Could you check a few things on this drawing? It's one solid part, dimensions in mm from its lowest x, y, z. Give positions to 0.01 mm unless a question says otherwise; leave off trailing zeros. Order: outer loops, then holes, each group sorted by start corner. A loop starts at its lowest first (then second) coordinate and runs counter-clockwise, first axis right, second up. Notation, with made-up numbers: M 85,18 L 103,18 A33 cw 103,56 Z; hole C 48,49.25 d7. An arc over 180 degrees is marked long. Use one line per item in the form item = value.
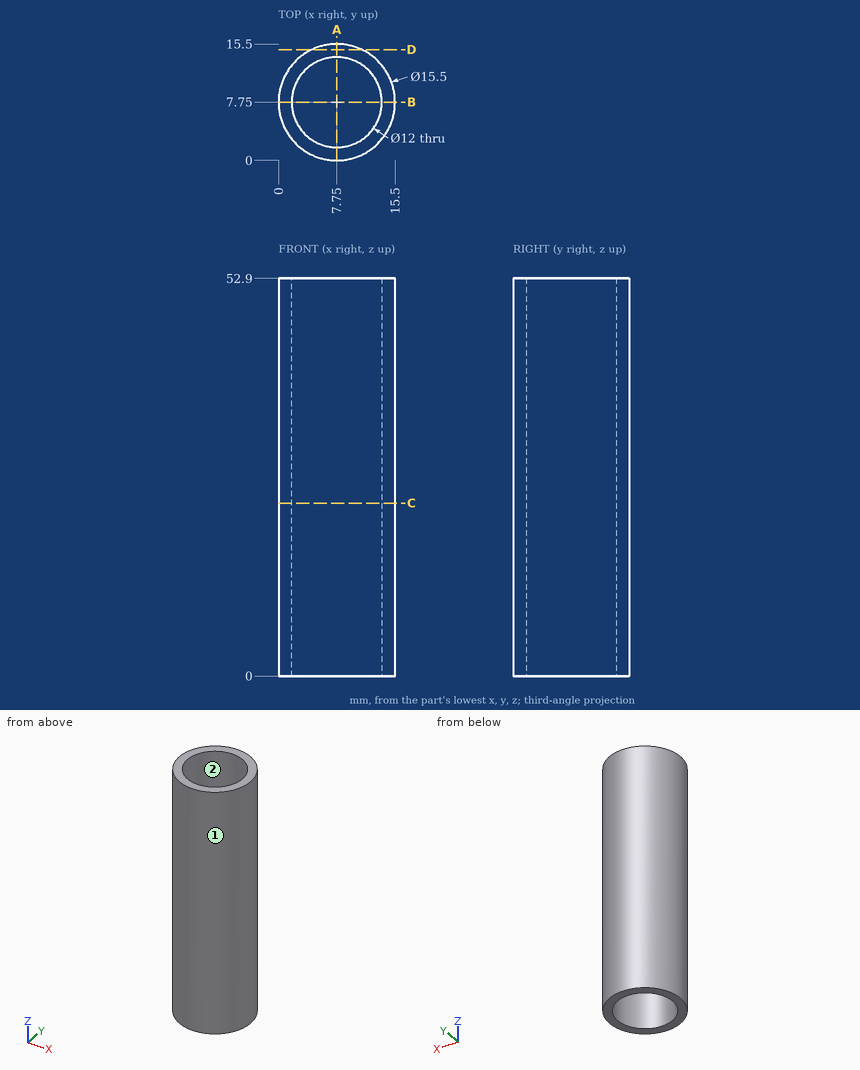
Q1. I want a section at C-C on z = 23. Write out the boundary of the cut face in (x, y).
Found:
outline = C 7.75,7.75 d15.5; hole C 7.75,7.75 d12
Q2. I want a section at D-D on y = 14.75. Write out the boundary of the cut face in (x, z), then the cut area to 3 significant figures.
Found:
outline = M 4.42,0 L 11.08,0 L 11.08,52.9 L 4.42,52.9 Z
area = 352 mm²
Q3. I need wall thicknesses on L1, parallel to Y at x = 7.75, z = 37; L2, parallel to X at y = 5, z = 26. Which ranges of each line are inside material? Lowest first, please.
Found:
L1 = 0 to 1.75, 13.75 to 15.5
L2 = 0.5 to 2.42, 13.08 to 15
Q4. Thinking about a two-plate mould opening in X: for the marked faces 1 and 2, which applies, +X half, -X half, draft (parallel to the pull), parting line (faces both ways), or undercut?
Found:
face_1 = parting line
face_2 = undercut
Q5. I'm going to push flat-ended pins straight in: pin 1 Ø1 at (y, z) = (5, 36) entering from -X; pin 2 Ø1 at (x, z) = (6, 26.5) entering from -Y; pin 3 Ø5 at (y, z) = (2.5, 13.5) entering from -X. Where does each tip first touch, or does it pass through?
Found:
pin_1 = 0.33
pin_2 = 0.1
pin_3 = 0.5
Q6. I want a section at A-A on x = 7.75. Write out the boundary of the cut face in (y, z), then the cut area to 3 significant figures.
Found:
outline = M 0,0 L 1.75,0 L 1.75,52.9 L 0,52.9 Z; M 13.75,0 L 15.5,0 L 15.5,52.9 L 13.75,52.9 Z
area = 185 mm²
